Source: CAD feature listing. Evaluate the final solid. Frame: model axes, mm. A direction names the side the tool comes from. Coordinates: 2 decimals unless noted, no trailing zeros. Order: outer loops, then holes, each group sorted by start corner. A loop starts at its lowest first (then second) coordinate and runs counter-clockwise, first axis right, second up. Notation, with made-up numbers: (-32.5, -38) - (5.5, -38) arc R14 cw to (5.5, -22) - close; hole circle Ø4 at (34, 84). An arc over 180 degrees is marked (long way). One line per question, with ' | ' between items.
Autodesk Inventor part; units mm, degrees
ref_plane "YZ Plane" through (0, 0, 0) normal (1, 0, 0) x (0, 1, 0)
ref_plane "XZ Plane" through (0, 0, 0) normal (0, 1, 0) x (-1, 0, 0)
ref_plane "XY Plane" through (0, 0, 0) normal (0, 0, 1) x (1, 0, 0)
sketch "Sketch1" plane through (0, 0, 0) normal (0, 1, 0) x (-1, 0, 0)
  line L0 (-10.105, -14.105) -> (10.105, -14.105)
  line L1 (14.105, -10.105) -> (14.105, 10.105)
  line L2 (10.105, 14.105) -> (-10.105, 14.105)
  line L3 (-14.105, 10.105) -> (-14.105, -10.105)
  line L4 (-14.105, -14.105) -> (14.105, 14.105) construction
  line L5 (14.105, -14.105) -> (-14.105, 14.105) construction
  arc A0 (14.105, 10.105) -> (10.105, 14.105) centre (10.105, 10.105) ccw
  arc A1 (-10.105, 14.105) -> (-14.105, 10.105) centre (-10.105, 10.105) ccw
  arc A2 (-14.105, -10.105) -> (-10.105, -14.105) centre (-10.105, -10.105) ccw
  arc A3 (10.105, -14.105) -> (14.105, -10.105) centre (10.105, -10.105) ccw
  line L6 (10.105, 14.105) -> (10.105, 8.105) construction
  line L7 (9.605, 8.105) -> (9.605, 2.105)
  line L8 (8.105, 9.605) -> (2.105, 9.605)
  line L9 (8.105, 9.605) -> (9.605, 8.105)
  line L10 (8.9013, 1.7376) -> (1.5695, 9.0695)
  line L11 (2.105, 9.605) -> (1.5695, 9.0695)
  line L12 (8.9013, 1.7376) -> (9.0695, 1.5695)
  line L13 (9.605, 2.105) -> (9.0695, 1.5695)
  line L14 (8.0814, 0.5776) -> (0.5776, 8.0814)
  line L15 (2.2082, 6.4508) -> (-8.8227, -4.58)
  line L16 (6.4508, 2.2082) -> (-4.58, -8.8227)
  line L17 (-4.58, -8.8227) -> (-7.58, -8.8227)
  line L18 (-8.8227, -4.58) -> (-8.8227, -7.58)
  line L19 (-8.8227, -7.58) -> (-7.58, -8.8227)
  line L20 (-10.105, 12.105) -> (10.105, 12.105)
  arc A4 (12.105, 10.105) -> (10.105, 12.105) centre (10.105, 10.105) ccw
  line L21 (12.105, 10.105) -> (12.105, -10.105)
  arc A5 (10.105, -12.105) -> (12.105, -10.105) centre (10.105, -10.105) ccw
  line L22 (10.105, -12.105) -> (-10.105, -12.105)
  arc A6 (-12.105, -10.105) -> (-10.105, -12.105) centre (-10.105, -10.105) ccw
  line L23 (-12.105, -10.105) -> (-12.105, 10.105)
  arc A7 (-10.105, 12.105) -> (-12.105, 10.105) centre (-10.105, 10.105) ccw
  point P0 (0, 0)
  point P1 (8.855, 8.855)
  point P2 (4.3295, 4.3295)
  dimension "d0" = 28.21
  dimension "d1" = 28.21
  dimension "d2" = 4
  dimension "d13" = 6
  dimension "d16" = 6
  dimension "d18" = 5
  dimension "d21" = 1.4
  dimension "d22" = 15.6
  dimension "d24" = 3
  dimension "d25" = 3
  dimension "d28" = 2
extrude "Extrusion5" add sketch "Sketch1" against normal blind 1.3 contours A2 L3 A1 L2 A0 L1 A3 L0
extrude "Extrusion6" add sketch "Sketch1" against normal blind 4 contours L20 A4 L21 A5 L22 A6 L23 A7
sketch "Sketch5" plane through (-2.2082, -4, 6.4508) normal (0.7071068, 0, -0.7071068) x (-0.7071068, 0, -0.7071068)
  line L0 (6, 0) -> (0, 0)
  line L1 (6, 0) -> (0, 0)
  line L2 (0, 0) -> (0, 0.5)
  line L3 (0, 0.5) -> (6, 0.5)
  line L4 (6, 0.5) -> (6, 0)
  point P0 (3, 4)
  dimension "d33" = 6
  dimension "d34" = 0.5
extrude "Extrusion7" cut sketch "Sketch5" against normal blind 4
sketch "Sketch6" plane through (0, 0, 0) normal (0, 1, 0) x (1, 0, 0)
  line L0 (-14.105, -14.105) -> (14.105, 14.105) construction
  line L1 (-14.105, 14.105) -> (14.105, -14.105) construction
  line L2 (-9.0695, -1.5695) -> (-1.5695, -9.0695)
  line L3 (2.8146, -11.4736) -> (11.2999, -2.9883)
  line L4 (1.1859, 7.1256) -> (-2.8423, 11.1538)
  line L5 (-2.8423, 11.1538) -> (-11.3275, 2.6685)
  line L6 (4.58, 8.8227) -> (7.58, 8.8227)
  line L7 (-6.4508, -2.2082) -> (4.58, 8.8227)
  line L8 (11.2999, -2.9883) -> (7.1256, 1.1859)
  line L9 (-2.2082, -6.4508) -> (-6.4508, -2.2082)
  line L10 (-2.2082, -6.4508) -> (2.8146, -11.4736)
  line L11 (-6.4508, -2.2082) -> (-11.3275, 2.6685)
  line L12 (8.8227, 4.58) -> (-2.2082, -6.4508)
  line L13 (7.1256, 1.1859) -> (6.9842, 1.3273)
  line L14 (1.1859, 7.1256) -> (1.3273, 6.9842)
  line L15 (6.2771, 2.0344) -> (-2.2082, -6.4508)
  line L16 (2.0344, 6.2771) -> (-6.4508, -2.2082)
  line L17 (6.9842, 1.3273) -> (6.2771, 2.0344)
  line L18 (1.3273, 6.9842) -> (2.0344, 6.2771)
  point P0 (0, 0)
  dimension "d39" = 20
  dimension "d53" = 12
extrude "Extrusion8" cut sketch "Sketch6" against normal through all
sketch "Sketch8" plane through (11.2999, -4, 2.9883) normal (-0.7071068, 0, 0.7071068) x (0.7071068, 0, 0.7071068)
  line L0 (0, 0) -> (-7.1033, 0)
  line L1 (0, 4) -> (0, 0)
  line L2 (0, 4) -> (0, 0)
  line L3 (0, 0) -> (-7.1033, 0)
  line L4 (-20, 4) -> (-20, 0)
  line L5 (-20, 4) -> (-20, 0)
  line L6 (-13.1033, 0) -> (-20, 0)
  line L7 (-13.0928, 0) -> (-20, 0)
  line L8 (-13.1033, 0) -> (-13.1033, 0.5)
  line L9 (-13.1033, 4) -> (-13.1033, 0)
  line L10 (-13.1033, 0.5) -> (-20, 4)
  line L11 (-7.1033, 0) -> (-7.1033, 0.5)
  line L12 (-7.1033, 0.5) -> (0, 4)
  point P0 (-10.1033, 4)
  point P1 (-13.1033, 0)
  dimension "d48" = 0.5
  dimension "d49" = 0.5
extrude "Extrusion10" add sketch "Sketch8" along normal blind 12
fillet "Fillet2" radius 1.5 2 edges at (2.0344, -1.75, -6.2771) (6.2771, -1.75, -2.0344)
properties part number "pieza_edu_fisica"
(1) Cut plane D-D (z = 6). Return the cut outline in (x, y) (3 decimals), and give its area (3 significant figures).
Taken from the geometry:
outline: (-14.105, -1.3) - (-12.105, -1.3) - (-12.105, -4) - (-9.605, -4) - (-9.605, 0) - (-14.105, 0) - close; (-4.639, -3.5) - (-2.659, -3.5) - (-2.659, 0) - (-4.639, 0) - close; (-1.757, -4) - (12.105, -4) - (12.105, -1.3) - (14.105, -1.3) - (14.105, 0) - (8.288, 0) - (-1.757, -3.5) - close | area: 60.0 mm²
(2) Cut plane C-C (y = -2). State how many separate pieces and enclosed holes the cut face has, and give its area (3 significant figures).
Taken from the geometry:
separate pieces: 1 | enclosed holes: 2 | area: 373 mm²
(3) Pull-direction query (X, two-part tool) for faces 1 (the flat face through (0, -3, 12.105)), 2 (the cylindrical face through (-11.535, -2.631, 11.504)), 3 (the flat face through (-5, -2, 9.605)); classes: pulls with the +X half, pulls with the -X half, needs draft (parallel to the pull), parting line crosses it, or undercut.
Taken from the geometry:
face 1: needs draft | face 2: pulls with the -X half | face 3: undercut
(4) Material intervals for L1, parallel to X at y = -3.6, z = -9.5 (3 decimals); L2, parallel to X at y = -3.65, z = 7.5 (3 decimals); L3, parallel to X at y = -1.05, z = 1 (3 decimals), sorted ascending. Write a range as from..to.
Taken from the geometry:
L1: x = -12.105..12.105 | L2: x = -12.105..-9.605, -3.139..12.105 | L3: x = -14.105..-7.659, 9.312..14.105
(5) Cut plane A-A (z = 1). Return the cut outline in (x, y) (1 decimal).
Taken from the geometry:
outline: (-14.1, -1.3) - (-12.1, -1.3) - (-12.1, -4) - (-5.2, -4) - (-5.2, -3.5) - (-7.7, -2.6) - (-7.7, 0) - (-14.1, 0) - close; (3.2, -4) - (12.1, -4) - (12.1, -1.3) - (14.1, -1.3) - (14.1, 0) - (9.3, 0) - (9.3, -1.4) - (3.2, -3.5) - close
(6) Set-up query: faces 4 (the flat face through (-12.105, -3, 0)), 5 (the flat face through (-5.08, -1.77, -3.98)), 6 (the flat face through (8.2, -2, -8.2)). Return all of +Z, -Z, +X, -X, +Y, -Y with unobstructed straight access to the full face (end or side cutting, diameter ignored); none if empty.
Taken from the geometry:
face 4: +Z, -Z, -X, -Y | face 5: +Y | face 6: +Y, -Y
(7) Pin query (flat end, axial travel): P1, Ø1.2, axis at x = -5.5, y = -1.5, coming from the -Z side (3 decimals); P2, Ø4, axis at x = -5, z = 4, coming from the -Y side; P3, Ø2, axis at x = 3, z = 7, coming from the +Y side; P4, Ø1.4, axis at y = -3, z = 3.5, coming from the -X side (3 decimals). Return the tip coordinate at first contact, or that it passes through.
Taken from the geometry:
P1: stops at z = -14.105 | P2: stops at y = -3.5 | P3: stops at y = -1 | P4: stops at x = -12.105
(8) Cut plane B-B (x = -8.5). Return the cut outline in (y, z) (3 decimals), and give its area (3 significant figures).
Taken from the geometry:
outline: (-4, -12.105) - (-1.3, -12.105) - (-1.3, -14.105) - (0, -14.105) - (0, -5.496) - (-2.029, 0.159) - (0, 0.159) - (0, 2.139) - (-4, 2.139) - close; (-4, 9.21) - (0, 9.21) - (0, 14.105) - (-1.3, 14.105) - (-1.3, 12.105) - (-4, 12.105) - close | area: 68.0 mm²
